Source: CAD feature listing. Evaluate the final solid. Frame: model axes, mm. A direction names the side the tool comes from. Round coordinates to 2 decimals unless told otherwise and drop trailing zeros. Write each loop counter-clockwise with the first axis right and the second up, starting at its lowest first coordinate (ties: lowest second). Pieces come first, ordered by that corner, then holes. Notation, with made-up numbers: M 26.25,2 L 69.25,2 A19 cw 69.25,14 Z; hole C 84,40.25 d5. An arc over 180 degrees is marked long. Use a Markdown table: item, result.
```python
from build123d import *

# Parameters (mm, degrees)
F1_DEPTH = 877
F3_DEPTH = 406.4


with BuildPart() as f1:
    # F0 (on Front) → F1 (new body)
    with BuildSketch(Plane.XZ):
        Polygon((-200.083994, 140.112044), (-200.083994, -204.083866), (206.316006, -204.083866), (206.316006, 140.112044), (155.516006, 190.912044), (-149.283994, 190.912044), align=None)
    extrude(amount=F1_DEPTH)

    # F2 (on face) → F3 (join)
    with BuildSketch(Plane.XZ.offset(877)):
        Polygon((-250.883994, 405.516134), (-250.883994, -204.083866), (-200.083994, -204.083866), (-200.083994, 140.112044), (-149.283994, 190.912044), (155.516006, 190.912044), (206.316006, 140.112044), (206.316006, -204.083866), (257.116006, -204.083866), (257.116006, 405.516134), (206.316006, 456.316134), (-200.083994, 456.316134), align=None)
    extrude(amount=-F3_DEPTH)


solid = f1.part
```
Q1. Reachability of faces 1 (the flat face through (-174.328, -232.006, 165.868)), 2 (the flat face through (181.27, -232.01, 165.16)), 3 (the flat face through (206.316, -232, -34)), 4 (the flat face through (5, -232, 190.912)), 5 (the flat face through (-200.084, -232, -30)) from +Z, -Z, +X, -X, +Y, -Y: full face, straight path, thin tool, end or side. Return the list, or none.
Results are:
| item | result |
|---|---|
| face 1 | +Z, -X, +Y |
| face 2 | +Z, +X, +Y |
| face 3 | +Z, -Z, +X, +Y |
| face 4 | +Z, +X, -X, +Y |
| face 5 | +Z, -Z, -X, +Y |
Q2. Section C-C on y = -284. Return loops of the section in (x, z).
Results are:
| item | result |
|---|---|
| outline | M -200.08,-204.08 L 206.32,-204.08 L 206.32,140.11 L 155.52,190.91 L -149.28,190.91 L -200.08,140.11 Z |
Q3. First-contact query: pin 1 Ø1.5 at (x, y) = (202, -196.5) entering from +Z; pin 2 Ø6 at (x, y) = (-76, -203.5) entering from +Z. Flat tips, straight axial feed; report the tip coordinate or a pass-through.
Results are:
| item | result |
|---|---|
| pin 1 | z = 145.18 |
| pin 2 | z = 190.91 |
Q4. Section A-A on z = -145. Return loops of the section in (x, y).
Results are:
| item | result |
|---|---|
| outline | M -250.88,-877 L 257.12,-877 L 257.12,-470.6 L 206.32,-470.6 L 206.32,0 L -200.08,0 L -200.08,-470.6 L -250.88,-470.6 Z |
Q5. Section B-B on x = -37.5. Return loops of the section in (y, z), plus the area to 3 significant figures.
Results are:
| item | result |
|---|---|
| outline | M -877,-204.08 L 0,-204.08 L 0,190.91 L -470.6,190.91 L -470.6,456.32 L -877,456.32 Z |
| area | 454,000 mm^2 |
Q6. Section D-D on z = 360. Return loops of the section in (x, y), plus the area to 3 significant figures.
Results are:
| item | result |
|---|---|
| outline | M -250.88,-877 L 257.12,-877 L 257.12,-470.6 L -250.88,-470.6 Z |
| area | 206,000 mm^2 |
Q7. Line query: L1, parallel to Z at x = 54.5, y = -296.5; L2, parallel to Y at x = 111, z = 359.5; L3, parallel to X at y = -108.5, z = 44. Output: solid intervals per line, ascending.
Results are:
| item | result |
|---|---|
| L1 | -204.08 to 190.91 |
| L2 | -877 to -470.6 |
| L3 | -200.08 to 206.32 |
